from build123d import *

# Parameters (mm, degrees)
PADR_OCIRCULAR1_COUNT = 4
FILETE1_R             = 0.5


with BuildPart() as part:
    # Esboço1 → Revolução1 (revolve)
    with BuildSketch(Plane(origin=(0, 0, 0), x_dir=(0, 0, -1), z_dir=(1, 0, 0)), mode=Mode.PRIVATE) as revolu_o1_sk:
        Polygon((0, 17.5), (0, 21.5), (-0.5, 21.5), (-0.5, 22), (0, 22), (0, 25.5), (-0.5, 25.5), (-0.5, 26), (0, 26), (0, 41), (-10, 41), (-10, 26), (-70, 26), (-70, 22), (-69.5, 22), (-69.5, 21.5), (-70, 21.5), (-70, 17.5), align=None)
    revolve(revolu_o1_sk.sketch.rotate(Axis((0, 0, 0), (0, 0, 1)), 90), axis=Axis((0, 0, 0), (0, 0, 1)))  # turned: the seam where the file's is

    # Esboço5 → Corte-Revolução1 (revolve, cut)
    with BuildSketch(Plane(origin=(0, 0, 0), x_dir=(0, 0, -1), z_dir=(1, 0, 0)), mode=Mode.PRIVATE) as corte_revolu_o1_sk:
        Polygon((0, 39), (-6.1, 39), (-6.1, 36.8), (-10, 36.8), (-10, 33.5), (0, 33.5), align=None)
    corte_revolu_o1 = revolve(corte_revolu_o1_sk.sketch.rotate(Axis((0, 33.5, 0), (0, 0, -1)), 180), axis=Axis((0, 33.5, 0), (0, 0, -1)), mode=Mode.SUBTRACT)  # turned: the seam where the file's is

    # PadrãoCircular1: Corte-Revolução1 ×4 about axis
    padr_ocircular1_axis = Axis((0, 0, 0), (0, 0, 1))
    for i in range(1, PADR_OCIRCULAR1_COUNT):
        add(corte_revolu_o1.rotate(padr_ocircular1_axis, i * 360 / PADR_OCIRCULAR1_COUNT), mode=Mode.SUBTRACT)

    # Filete1
    filete1_edges = [part.edges().sort_by_distance(p)[0] for p in [
        (26, 0, 70),
        (41, 0, 10),
        (41, 0, 0),
    ]]
    fillet(filete1_edges, radius=FILETE1_R)


solid = part.part
Could you check a few things on this model? Use its own coordinates, in mm. A direction names the side the tool comes from. Give positions to 0.01 mm unless a question says otherwise; leave off trailing zeros. Order: outer loops, then holes, each group sorted by start corner. A loop starts at its lowest first (then second) coordinate and runs counter-clockwise, first axis right, second up.
1. Will these pins go through, and if not, where does the flat tip stop? P1, Ø1, axis at x = 13.5, z = 21, coming from the -Y side; P2, Ø7.5, axis at x = 33.5, y = 0, coming from the +Z side; P3, Ø3, axis at y = 18, z = 57, coming from the +X side; P4, Ø17.5, axis at x = -33.5, y = 0, coming from the +Z side.
2. Suppose I cut it at B-B (z = 12.5). List the corners of the cut face in (x, y) for me, plus the area to 3 significant figures.
3. I need wall thicknesses on L1, parallel to Y at x = -6.5, z = 59; L2, parallel to Y at x = 4, z = 65; L3, parallel to X at y = 33, z = 3. Which ranges of each line are inside material? Lowest first, please.
4. Suppose I cut it at A-A (z = 5). List the corners of the cut face in (x, y) for me, plus the area to 3 significant figures.
5. Suppose I cut it at C-C (y = 1.5). Give the number of separate pieces and of enclosed holes in the cut face, plus the area to 3 significant figures.
6. We'd pull the mould along Y, two halves only. Please class faces 4 (the cylindrical face through (-37.874, 15.703, 5.063)), 5 (the flat face through (0.6, 26.4, 10)), 6 (the cylindrical face through (4.769, 21.477, 69.746)): pulls with the +Y half, pulls with the -Y half, needs draft (parallel to the pull), parting line crosses it, or undercut.
7. For faces 1 (the flat face through (-20.9, 7.4, 0)), 2 (the cylindrical face through (2.799, -21.317, 69.754)), 3 (the flat face through (17.2, 19.1, 0.5)), which set-ups out of +Z, -Z, +X, -X, +Y, -Y let a thin tool reach every point of the face, with its end or its side?
Solved:
1. P1: stops at y = -22.52
1. P2: stops at z = 10
1. P3: stops at x = 20.09
1. P4: stops at z = 70
2. outline: circle Ø52 at (0, 0); hole circle Ø35 at (0, 0)
2. area: 1,160 mm2
3. L1: y = -25.17 to -16.25, 16.25 to 25.17
3. L2: y = -25.69 to -17.04, 17.04 to 25.69
3. L3: x = -24.33 to -5.48, 5.48 to 24.33
4. outline: circle Ø82 at (0, 0); hole circle Ø11 at (-33.5, 0); hole circle Ø35 at (0, 0); hole circle Ø11 at (0, -33.5); hole circle Ø11 at (0, 33.5); hole circle Ø11 at (33.5, 0)
4. area: 3,940 mm2
5. separate pieces: 4
5. enclosed holes: 0
5. area: 1,320 mm2
6. face 4: parting line crosses it
6. face 5: needs draft
6. face 6: undercut
7. face 1: -Z, +X, -X, +Y, -Y
7. face 2: +Z
7. face 3: -Z
